from build123d import *

# Parameters (mm, degrees)
G1_4_GEWINDEBOHRUNG1_D          = 11.445
G1_4_GEWINDEBOHRUNG1_DEPTH      = 100
SKIZZE6_R                       = 8
SCHNITT_LINEAR_AUSTRAGEN1_DEPTH = 9.75
SKIZZE7_R                       = 5
SCHNITT_LINEAR_AUSTRAGEN2_DEPTH = 30
KREISMUSTER1_COUNT              = 3
KREISMUSTER1_ANGLE              = 180


with BuildPart() as part:
    # Skizze1 → Rotation1 (revolve)
    with BuildSketch(Plane.XY):
        Polygon((0, 17.25), (0, 32.5), (100, 32.5), (100, 1.5), (85, 1.5), (76.625576451, 17.25), align=None)
    revolve(axis=Axis((0, 0, 0), (1, 0, 0)))

    # G1/4 Gewindebohrung1
    with Locations(Plane(origin=(100, 0, 0), x_dir=(0, 0, 1), z_dir=(1, 0, 0))):
        with Locations((0, 0)):
            Hole(G1_4_GEWINDEBOHRUNG1_D / 2, depth=G1_4_GEWINDEBOHRUNG1_DEPTH)

    # Skizze6 → Schnitt-Linear austragen1 (cut)
    with BuildSketch(Plane.XY.offset(32.5)):
        with Locations((50, 0)):
            Circle(SKIZZE6_R)
    schnitt_linear_austragen1 = extrude(amount=-SCHNITT_LINEAR_AUSTRAGEN1_DEPTH, mode=Mode.SUBTRACT)

    # Skizze7 → Schnitt-Linear austragen2 (cut)
    with BuildSketch(Plane.XY.offset(32.5)):
        with Locations((50, 0)):
            Circle(SKIZZE7_R)
    schnitt_linear_austragen2 = extrude(amount=-SCHNITT_LINEAR_AUSTRAGEN2_DEPTH, mode=Mode.SUBTRACT)

    # Kreismuster1: Schnitt-Linear austragen1, Schnitt-Linear austragen2 ×3 about axis
    kreismuster1_axis = Axis((0, 0, 0), (-1, 0, 0))
    for i in range(1, KREISMUSTER1_COUNT):
        add(schnitt_linear_austragen1.rotate(kreismuster1_axis, i * KREISMUSTER1_ANGLE / (KREISMUSTER1_COUNT - 1)), mode=Mode.SUBTRACT)
        add(schnitt_linear_austragen2.rotate(kreismuster1_axis, i * KREISMUSTER1_ANGLE / (KREISMUSTER1_COUNT - 1)), mode=Mode.SUBTRACT)


solid = part.part
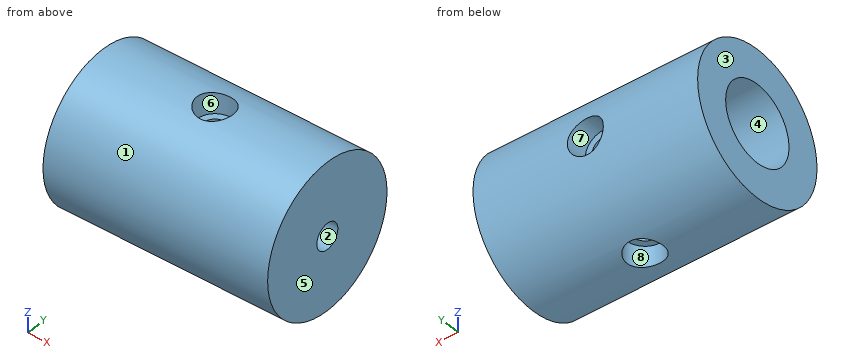
For this review, take the finished solid that the model builds, in its own axes (mm). Face numbers are marked on the shaded views. A direction names the side the tool comes from. Give positions to 0.01 mm unless a question says otherwise; leave off trailing zeros. Order: outer loops, then holes, each group sorted by start corner. A loop starts at its lowest first (then second) coordinate and runs counter-clockwise, first axis right, second up. Notation, with made-up numbers: (48.5, 34) -> (54.5, 34) arc R23 ccw to (54.5, 70) -> close; hole circle Ø7 at (-9, 61). An arc over 180 degrees is marked (long way). Write item = value, one per line.
1) We need section D-D, the plane z = -27.5. Give the boundary of the cut face in (x, y), and give its area (3 significant figures).
Findings:
outline = (0, -17.32) -> (100, -17.32) -> (100, 17.32) -> (0, 17.32) -> close; hole circle Ø16 at (50, 0)
area = 3,260 mm^2
2) Draft analysis for pull direction Z (two halves, no side actions). For the marked faces 1, 2, 3 and 4, state which applies: pulls with the +Z half, pulls with the -Z half, needs draft (parallel to the pull), parting line crosses it, or undercut.
Findings:
face_1 = parting line crosses it
face_2 = undercut
face_3 = needs draft
face_4 = undercut
3) For the marked faces 5, 6, 7 and 8, list the 3-axis set-ups (+Z, -Z, +X, -X, +Y, -Y) from which the entire face can be reached by the end or side of a thin tool; tool diameter is ignored.
Findings:
face_5 = +Z, -Z, +X, +Y, -Y
face_6 = +Z
face_7 = +Y
face_8 = -Z
4) We need section B-B, the plane z = 0. Give the boundary of the cut face in (x, y), and give its area (3 significant figures).
Findings:
outline = (0, -32.5) -> (100, -32.5) -> (100, -5.72) -> (82.75, -5.72) -> (76.63, -17.25) -> (0, -17.25) -> close; (0, 17.25) -> (45, 17.25) -> (45, 22.75) -> (42, 22.75) -> (42, 32.5) -> (0, 32.5) -> close; (55, 17.25) -> (76.63, 17.25) -> (82.75, 5.72) -> (100, 5.72) -> (100, 32.5) -> (58, 32.5) -> (58, 22.75) -> (55, 22.75) -> close
area = 3,310 mm^2
5) We need section C-C, the plane x = 50. Give the boundary of the cut face in (y, z), and give its area (3 significant figures).
Findings:
outline = (-8, -31.5) -> (-8, -22.75) -> (-5, -22.75) -> (-5, -16.51) arc R17.25 cw to (-5, 16.51) -> (-5, 22.75) -> (-8, 22.75) -> (-8, 31.5) arc R32.5 ccw to start; (5, -22.75) -> (8, -22.75) -> (8, -31.5) arc R32.5 ccw to (31.5, -8) -> (22.75, -8) -> (22.75, -5) -> (16.51, -5) arc R17.25 cw to (5, -16.51) -> close; (5, 16.51) arc R17.25 cw to (16.51, 5) -> (22.75, 5) -> (22.75, 8) -> (31.5, 8) arc R32.5 ccw to (8, 31.5) -> (8, 22.75) -> (5, 22.75) -> close
area = 1,760 mm^2
6) To check wall thickness, follow L1, parallel to X at y = 0, z = 27.25; L2, parallel to Y at x = 50, z = -27; L3, parallel to Y at x = 39, z = 10. State the ranges of each line that lie inside material, in increasing order. Write a range as from..to.
Findings:
L1 = 0..42, 58..100
L2 = -18.09..-8, 8..18.09
L3 = -30.92..-14.06, 14.06..30.92
7) Insertion check: pin 1 (5 mm diameter, centred on x = 64.5, z = 8.5, fed in from +Y); pin 2 (10 mm diameter, centred on x = 11.5, y = 22, fed in from -Z); pin 3 (1 mm diameter, centred on x = 90, y = -13, fed in from -Z). Each pin has a flat end and moves straight along its axis. Give the tip position at first contact, or say it passes through.
Findings:
pin_1 = 31.94
pin_2 = -27.7
pin_3 = -30
8) We need section A-A, the plane y = 0. Give the boundary of the cut face in (x, z), and give its area (3 significant figures).
Findings:
outline = (0, -32.5) -> (42, -32.5) -> (42, -22.75) -> (45, -22.75) -> (45, -17.25) -> (0, -17.25) -> close; (0, 17.25) -> (45, 17.25) -> (45, 22.75) -> (42, 22.75) -> (42, 32.5) -> (0, 32.5) -> close; (55, -22.75) -> (58, -22.75) -> (58, -32.5) -> (100, -32.5) -> (100, -5.72) -> (82.75, -5.72) -> (76.63, -17.25) -> (55, -17.25) -> close; (55, 17.25) -> (76.63, 17.25) -> (82.75, 5.72) -> (100, 5.72) -> (100, 32.5) -> (58, 32.5) -> (58, 22.75) -> (55, 22.75) -> close
area = 3,100 mm^2
